```python
from build123d import *

# Parameters (mm, degrees)
SALIENTE_EXTRUIR1_DEPTH = 3


with BuildPart() as part:
    # Croquis1 → Saliente-Extruir1 (new body)
    with BuildSketch(Plane.XY):
        with BuildLine():
            Line((-144.434437963, 23.831289655), (-139.359958663, 23.831289655))
            Line((-139.359958663, 23.831289655), (-139.359958663, 21.081289655))
            Line((-139.359958663, 21.081289655), (-144.434437963, 21.081289655))
            Line((-144.434437963, 21.081289655), (-144.434437963, 15.568266464))
            ThreePointArc((-144.434437963, 15.568266464), (-144.212105673, 14.651807238), (-143.59454045, 13.93910649))
            ThreePointArc((-143.59454045, 13.93910649), (-141.78704859, 13.000742202), (-139.79067514, 12.598191072))
            ThreePointArc((-139.79067514, 12.598191072), (-138.731334246, 12.648248724), (-137.706379935, 12.920604299))
            add(Edge.make_bspline(
                [(-137.706379935, 12.920604299), (-112.690499862, 22.507679551), (-138.413124465, 31.087686647)],
                knots=[5.204835954, 5.204835954, 5.204835954, 7.417095332, 7.417095332, 7.417095332], degree=2, weights=[1, 0.44812481, 1]))
            ThreePointArc((-138.413124465, 31.087686647), (-139.809326003, 31.341133977), (-141.220500745, 31.192136898))
            ThreePointArc((-141.220500745, 31.192136898), (-142.419935003, 30.779687584), (-143.533969481, 30.173317932))
            ThreePointArc((-143.533969481, 30.173317932), (-144.194986604, 29.451610375), (-144.434437963, 28.502680197))
            Line((-144.434437963, 28.502680197), (-144.434437963, 23.831289655))
        make_face()
    extrude(amount=SALIENTE_EXTRUIR1_DEPTH)


solid = part.part
```
For this review, take the finished solid that the model builds, in its own axes (mm). A direction names the side the tool comes from. Coordinates: 2 decimals unless noted, no trailing zeros. Loops run counter-clockwise (first coordinate to the right, second up) from the corner with the lowest first, then second, coordinate; pieces in that order, holes last.
1. Mouldability with a two-part tool opening along Y and no side actions: class faces 1 (the flat face through (-142, 23.831, 1)), 2 (the cylindrical face through (-142.4, 30.79, 1.48)), 3 (the cylindrical face through (-138.746, 12.646, 1.479)), 4 (the flat face through (-139.36, 22, 1)) as +Y half, -Y half, draft (parallel to the pull), parting line (faces both ways), or undercut.
2. For line 1 (Y direction, x = -142.25, z = 1.85); line 2 (Y direction, x = -139.75, z = 0.6); line 3 (X direction, y = 22, z = 0.8), list the stretches that pass through material, from the lowest coordinate up.
3. Insertion check: P1, Ø1.4, axis at y = 23, z = 1.5, coming from the -X side; P2, Ø1.5, axis at x = -140.5, z = 2.5, coming from the -Y side. Each pin has a flat end and moves straight along its axis. Give the tip position at first contact, or say it passes through.
4. For faces 5 (the flat face through (-142, 21.081, 1)), 6 (the flat face through (-138, 21, 0)), list the 3-axis set-ups (+Z, -Z, +X, -X, +Y, -Y) from which the entire face can be reached by the end or side of a thin tool; tool diameter is ignored.
5. Add section A-A, the plane x = -142.5. Give the boundary of the cut face in (y, z).
Result:
1. face 1: undercut
1. face 2: +Y half
1. face 3: -Y half
1. face 4: undercut
2. line 1: y = 13.18 to 21.08, 23.83 to 30.85
2. line 2: y = 12.6 to 21.08, 23.83 to 31.34
2. line 3: x = -139.36 to -130.2
3. P1: stops at x = -139.36
3. P2: stops at y = 12.6
4. face 5: +Z, -Z, -X
4. face 6: -Z, +X, -X, +Y, -Y
5. outline: (13.3, 0) - (21.08, 0) - (21.08, 3) - (13.3, 3) - close; (23.83, 0) - (30.74, 0) - (30.74, 3) - (23.83, 3) - close
